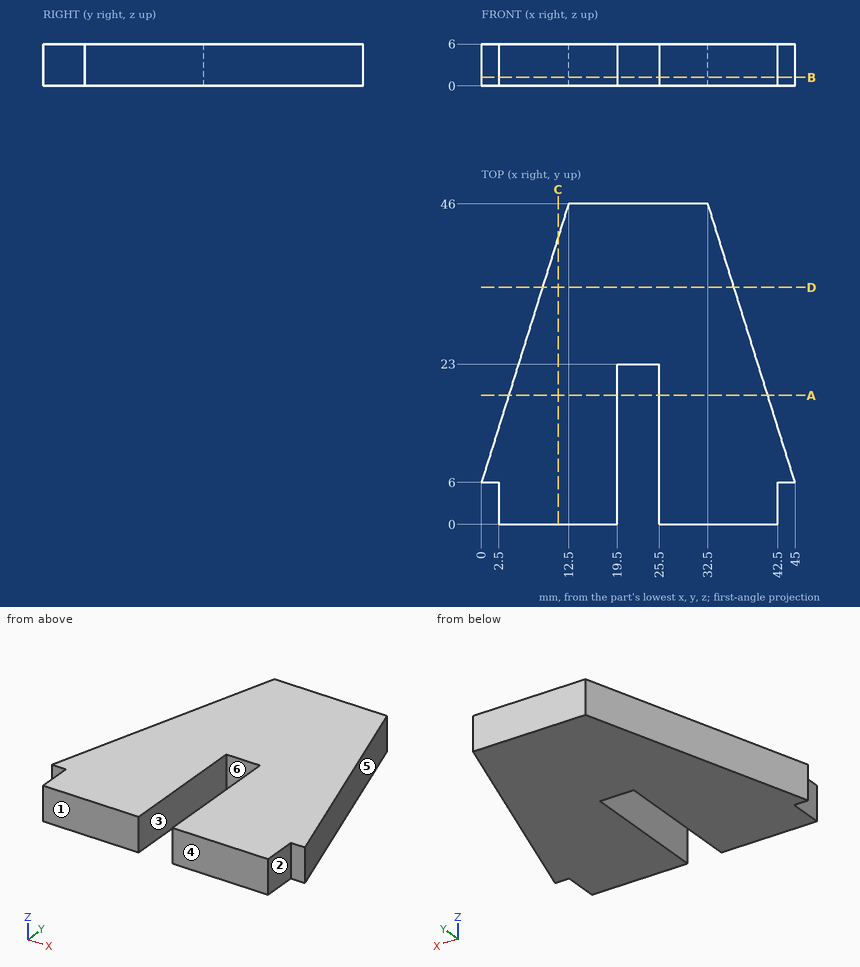
Could you check a few things on this drawing? It's one solid part, dimensions in mm from its lowest x, y, z. A direction names the side the tool comes from. Round coordinates to 2 decimals unless told otherwise and drop trailing zeros. Order: outer loops, then holes, each group sorted by start corner. A loop starts at its lowest first (then second) coordinate and runs counter-clockwise, first axis right, second up. Notation, with made-up numbers: M 81,67.25 L 104,67.25 A15 cw 104,88.25 Z; hole C 23,28.5 d8. An arc over 180 degrees is marked long. One line per question, with ' | ' between items.
1) Imagine slicing it at D-D, the plane y = 34. Write out the boundary of the cut face in (x, z).
Checked values:
outline: M 8.75,0 L 36.25,0 L 36.25,6 L 8.75,6 Z
2) I'm going to push flat-ended pins straight in: pin 1 Ø10 at (x, y) = (35, 20) entering from -Z; pin 2 Ø1.8 at (y, z) = (16, 2.5) entering from +X; pin 3 Ø3 at (y, z) = (2, 1.5) entering from -X; pin 4 Ø1.8 at (y, z) = (3, 2.5) entering from +X. Where does each tip first touch, or does it pass through?
Checked values:
pin 1: stops at z = 0 | pin 2: stops at x = 42.16 | pin 3: stops at x = 2.5 | pin 4: stops at x = 42.5
3) Imagine slicing it at B-B, the plane z = 1.2. Write out the boundary of the cut face in (x, y).
Checked values:
outline: M 0,6 L 2.5,6 L 2.5,0 L 19.5,0 L 19.5,23 L 25.5,23 L 25.5,0 L 42.5,0 L 42.5,6 L 45,6 L 32.5,46 L 12.5,46 Z
4) We'd pull the mould along X, two halves only. Please class the marked faces 4, 5 and 6: released by +X, released by -X, zero draft, split by the parting line, or undercut.
Checked values:
face 4: zero draft | face 5: released by +X | face 6: undercut
5) Imagine slicing it at A-A, the plane y = 18.5. Write out the boundary of the cut face in (x, z), plus the area to 3 significant figures.
Checked values:
outline: M 3.91,0 L 19.5,0 L 19.5,6 L 3.91,6 Z; M 25.5,0 L 41.09,0 L 41.09,6 L 25.5,6 Z | area: 187 mm²
6) Imagine slicing it at C-C, the plane x = 11. Write out the boundary of the cut face in (y, z), plus the area to 3 significant figures.
Checked values:
outline: M 0,0 L 41.2,0 L 41.2,6 L 0,6 Z | area: 247 mm²
7) I need wall thicknesses on line 1 (X direction, y = 3, z = 4.4); line 2 (X direction, y = 20, z = 3.2) (3 decimals); line 3 (Y direction, x = 23.5, z = 2.8). Which ranges of each line are inside material? Lowest first, please.
Checked values:
line 1: x = 2.5 to 19.5, 25.5 to 42.5 | line 2: x = 4.375 to 19.5, 25.5 to 40.625 | line 3: y = 23 to 46
8) On a 3-axis mill with a long thin cutter (end or side, diameter ignored), from which of +Z, -Z, +X, -X, +Y, -Y can I reach the whole of each face in a straight line? I mean the marked faces 1, 2 and 3. Say none if no direction works.
Checked values:
face 1: +Z, -Z, +X, -X, -Y | face 2: +Z, -Z, +X, -Y | face 3: +Z, -Z, -Y
